```python
from build123d import *

# Parameters (mm, degrees)
SKETCH1_W           = 80
SKETCH1_H           = 45
BOSS_EXTRUDE1_DEPTH = 42
SKETCH3_W           = 22
SKETCH3_H           = 28
CUT_EXTRUDE2_DEPTH  = 46
SKETCH4_W           = 10
SKETCH4_H           = 17
CUT_EXTRUDE3_DEPTH  = 28
SKETCH7_R           = 11.5
CUT_EXTRUDE5_DEPTH  = 3.5
SKETCH11_R          = 1.75
CUT_EXTRUDE6_DEPTH  = 10
SKETCH12_R          = 5
CUT_EXTRUDE7_DEPTH  = 42.5
SKETCH13_R          = 7.5
CUT_EXTRUDE8_DEPTH  = 46
SKETCH14_W          = 12.099538741
SKETCH14_H          = 10
CUT_EXTRUDE9_DEPTH  = 46
SKETCH15_R          = 1.712332533
CUT_EXTRUDE10_DEPTH = 43
SKETCH16_R          = 1.85
CUT_EXTRUDE11_DEPTH = 8
FILLET2_R           = 5


with BuildPart() as part:
    # Sketch1 → Boss-Extrude1 (new body)
    with BuildSketch(Plane.XY):
        with Locations((40, 22.5)):
            Rectangle(SKETCH1_W, SKETCH1_H)
    extrude(amount=BOSS_EXTRUDE1_DEPTH)

    # Sketch3 → Cut-Extrude2 (cut, through all)
    with BuildSketch(Plane(origin=(0, 45, 0), x_dir=(1, 0, 0), z_dir=(0, 1, 0))):
        with Locations((11, -14)):
            Rectangle(SKETCH3_W, SKETCH3_H)
    extrude(amount=-CUT_EXTRUDE2_DEPTH, mode=Mode.SUBTRACT)

    # Sketch4 → Cut-Extrude3 (cut)
    with BuildSketch(Plane.ZY):
        with Locations((35, 22.5)):
            Rectangle(SKETCH4_W, SKETCH4_H)
    extrude(amount=-CUT_EXTRUDE3_DEPTH, mode=Mode.SUBTRACT)

    # Sketch7 → Cut-Extrude5 (cut)
    with BuildSketch(Plane(origin=(0, 45, 0), x_dir=(1, 0, 0), z_dir=(0, 1, 0))):
        with Locations((38, -21)):
            Circle(SKETCH7_R)
    extrude(amount=-CUT_EXTRUDE5_DEPTH, mode=Mode.SUBTRACT)

    # Sketch11 → Cut-Extrude6 (cut)
    with BuildSketch(Plane(origin=(0, 41.5, 0), x_dir=(1, 0, 0), z_dir=(0, 1, 0))):
        with Locations((32.201639679, -26.511716392)):
            Circle(SKETCH11_R)
        with Locations((32.488283608, -15.201639679)):
            Circle(SKETCH11_R)
        with Locations((43.798360321, -15.488283608)):
            Circle(SKETCH11_R)
        with Locations((43.511716392, -26.798360321)):
            Circle(SKETCH11_R)
    extrude(amount=-CUT_EXTRUDE6_DEPTH, mode=Mode.SUBTRACT)

    # Sketch12 → Cut-Extrude7 (cut, through all)
    with BuildSketch(Plane(origin=(0, 41.5, 0), x_dir=(1, 0, 0), z_dir=(0, 1, 0))):
        with Locations((38, -21)):
            Circle(SKETCH12_R)
    extrude(amount=-CUT_EXTRUDE7_DEPTH, mode=Mode.SUBTRACT)

    # Sketch13 → Cut-Extrude8 (cut, through all)
    with BuildSketch(Plane(origin=(0, 45, 0), x_dir=(1, 0, 0), z_dir=(0, 1, 0))):
        with Locations((68, -21)):
            Circle(SKETCH13_R)
    extrude(amount=-CUT_EXTRUDE8_DEPTH, mode=Mode.SUBTRACT)

    # Sketch14 → Cut-Extrude9 (cut, through all)
    with BuildSketch(Plane(origin=(0, 45, 0), x_dir=(1, 0, 0), z_dir=(0, 1, 0))):
        with Locations((73.950230629, -21)):
            Rectangle(SKETCH14_W, SKETCH14_H)
    extrude(amount=-CUT_EXTRUDE9_DEPTH, mode=Mode.SUBTRACT)

    # Sketch15 → Cut-Extrude10 (cut, through all)
    with BuildSketch(Plane.XY.offset(42)):
        with Locations((12.5, 22.500000001)):
            Circle(SKETCH15_R)
    extrude(amount=-CUT_EXTRUDE10_DEPTH, mode=Mode.SUBTRACT)

    # Sketch16 → Cut-Extrude11 (cut)
    with BuildSketch(Plane.XY.offset(42)):
        with Locations((10, 37.5)):
            Circle(SKETCH16_R)
        with Locations((70, 37.5)):
            Circle(SKETCH16_R)
        with Locations((70, 7.5)):
            Circle(SKETCH16_R)
        with Locations((10, 7.5)):
            Circle(SKETCH16_R)
    extrude(amount=-CUT_EXTRUDE11_DEPTH, mode=Mode.SUBTRACT)

    # Fillet2
    fillet2_edges = [part.edges().sort_by_distance(p)[0] for p in [
        (22, 22.5, 0),
        (22, 22.5, 28),
        (80, 22.5, 0),
    ]]
    fillet(fillet2_edges, radius=FILLET2_R)


solid = part.part
```
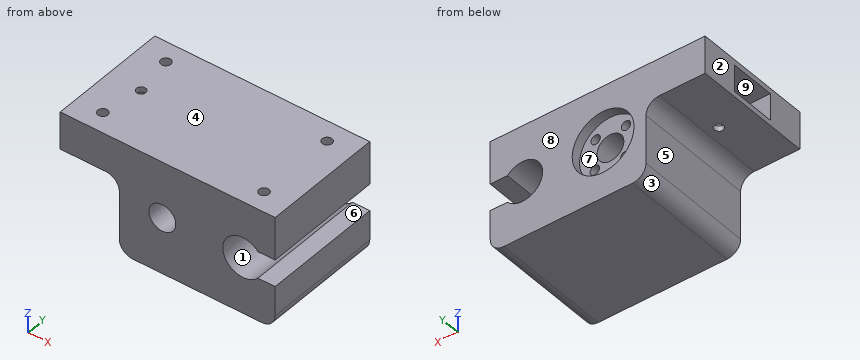
Here's how the part is built. I have some questions about the finished solid (model axes, mm). Face numbers are marked on the shaded views. A direction names the side the tool comes from. Round coordinates to 2 decimals unless told otherwise and drop trailing zeros. Loops run counter-clockwise (first coordinate to the right, second up) from the corner with the lowest first, then second, coordinate; pieces in that order, holes last. Notation, with made-up numbers: (41, -5) -> (56, -5) arc R24 cw to (56, 23) -> close; hole circle Ø7 at (5.5, 45.5). An arc over 180 degrees is marked (long way). Answer as CSV lines item,"result".
1. If we section it at D-D on z = 37: Please give me the cut outline in (x, y), plus the area to 3 significant figures.
Final values:
outline,"(0, 0) -> (80, 0) -> (80, 45) -> (0, 45) -> (0, 31) -> (28, 31) -> (28, 14) -> (0, 14) -> close; hole circle Ø3.7 at (10, 7.5); hole circle Ø3.7 at (10, 37.5); hole circle Ø3.7 at (70, 7.5); hole circle Ø3.7 at (70, 37.5)"
area,"3,080 mm^2"
2. If we section it at B-B on z = 21: Please give me the cut outline in (x, y), plus the area to 3 significant figures.
Final values:
outline,"(22, 0) -> (33, 0) -> (33, 41.5) -> (26.5, 41.5) -> (26.5, 45) -> (22, 45) -> close; (43, 0) -> (60.5, 0) -> (60.5, 45) -> (49.5, 45) -> (49.5, 41.5) -> (43, 41.5) -> close"
area,"1,240 mm^2"
3. If I drill on L1, parallel to Y at x = 10, z = 36.25; L2, parallel to Z at x = 14.5, y = 24; L3, parallel to Y at x = 13, z = 37.5, over which ranges is the centre line in solid material (lowest first)?
Final values:
L1,"y = 0 to 5.65, 9.35 to 14, 31 to 35.65, 39.35 to 45"
L2,"z = 28 to 30, 40 to 42"
L3,"y = 0 to 14, 31 to 45"
4. Thinking about a two-plate mould opening in Z: for the marked faces 1, 2, 3 and 4, which applies, released by +Z, released by -Z, zero draft, split by the parting line, or undercut?
Final values:
face 1,"undercut"
face 2,"zero draft"
face 3,"released by -Z"
face 4,"released by +Z"
5. For pin 1 (8 mm diameter, centred on y = 25, z = 16, fed in from -X); pin 2 (3 mm diameter, centred on x = 43, z = 15, fed in from +Y); pin 3 (2 mm diameter, centred on x = 10, y = 7.5, fed in from -Z), each with a flat end and sliding along its axis, tell me the tip position at first contact or that it passes through.
Final values:
pin 1,"stops at x = 22"
pin 2,"stops at y = 41.5"
pin 3,"stops at z = 28"
6. Which directions (+Z, -Z, +X, -X, +Y, -Y) give clear straight access to the entire face, cutting with the end or side of a thin tool? Please do the marked faces 5, 6, 7, 8 and 9.
Final values:
face 5,"-Z, -X, +Y, -Y"
face 6,"+X, +Y, -Y"
face 7,"+Y"
face 8,"+Z, -Z, +X, -X, +Y"
face 9,"-X"
7. If we section it at A-A on y = 22.5: Please give me the cut outline in (x, z), plus the area to 3 significant figures.
Final values:
outline,"(0, 28) -> (10.79, 28) -> (10.79, 30) -> (0, 30) -> close; (0, 40) -> (10.79, 40) -> (10.79, 42) -> (0, 42) -> close; (14.21, 28) -> (17, 28) arc R5 cw to (22, 23) -> (22, 5) arc R5 ccw to (27, 0) -> (75, 0) arc R5 ccw to (80, 5) -> (80, 16) -> (73.59, 16) arc R7.5 cw (long way) to (73.59, 26) -> (80, 26) -> (80, 42) -> (14.21, 42) -> (14.21, 40) -> (28, 40) -> (28, 30) -> (14.21, 30) -> close; hole circle Ø10 at (38, 21)"
area,"2,140 mm^2"
8. If we section it at C-C on y = 3.5: Please give me the cut outline in (x, z), plus the area to 3 significant figures.
Final values:
outline,"(0, 28) -> (17, 28) arc R5 cw to (22, 23) -> (22, 5) arc R5 ccw to (27, 0) -> (75, 0) arc R5 ccw to (80, 5) -> (80, 16) -> (73.59, 16) arc R7.5 cw (long way) to (73.59, 26) -> (80, 26) -> (80, 42) -> (0, 42) -> close; hole circle Ø10 at (38, 21)"
area,"2,430 mm^2"
